The model under review builds one solid part; all positions refer to its coordinate system, in mm. A direction names the side the tool comes from. Coordinates: 2 decimals unless noted, no trailing zeros. Loops run counter-clockwise (first coordinate to the right, second up) from the corner with the lowest first, then second, coordinate; pieces in that order, holes last. Notation, with made-up numbers: M 9.5,-2.75 L 18.5,-2.75 A22 cw 18.5,34.25 Z; hole C 9,23 d4. An arc over 180 degrees is marked long. Return JSON: item names as keys, results as strings.
```python
from build123d import *

# Parameters (mm, degrees)
FLANGE_BASE1_START             = -5
FLANGE_BASE1_OUTLINE_W         = 35
FLANGE_BASE1_OUTLINE_H         = 80
FLANGE_BASE1_DEPTH             = 10
FURO_ROSCADO_DE_M10X1_51_D     = 8.5
FURO_ROSCADO_DE_M10X1_51_DEPTH = 29.946342369
FURO_ROSCADO_DE_M10X1_51_TIP   = 2.553657631
ESBO_O9_R                      = 10
CORTE_EXTRUS_O2_DEPTH          = 3
CORTE_EXTRUS_O3_DEPTH          = 45.218208919


# Read off the part's stored shape, not the designer's step: Flange-base1
with BuildPart() as part:
    # Flange-base1 outline → Flange-base1 (new body)
    with BuildSketch(Plane.XY.offset(FLANGE_BASE1_START)):
        Rectangle(FLANGE_BASE1_OUTLINE_W, FLANGE_BASE1_OUTLINE_H)
    extrude(amount=FLANGE_BASE1_DEPTH)

    # Furo roscado de M10x1.51
    with Locations(Plane.XY.offset(5)):
        with Locations((0, 25)):
            Hole(FURO_ROSCADO_DE_M10X1_51_D / 2, depth=FURO_ROSCADO_DE_M10X1_51_DEPTH)
            with Locations((0, 0, -(FURO_ROSCADO_DE_M10X1_51_DEPTH + FURO_ROSCADO_DE_M10X1_51_TIP / 2))):  # 118° drill point
                Cone(0, FURO_ROSCADO_DE_M10X1_51_D / 2, FURO_ROSCADO_DE_M10X1_51_TIP, mode=Mode.SUBTRACT)

    # Esboço9 → Corte-extrusão2 (cut)
    with BuildSketch(Plane.XY.offset(5)):
        with Locations((0, -15)):
            Circle(ESBO_O9_R)
    extrude(amount=-CORTE_EXTRUS_O2_DEPTH, mode=Mode.SUBTRACT)

    # Esboço10 → Corte-extrusão3 (cut, through all)
    with BuildSketch(Plane.XY.offset(2)):
        with BuildLine():
            Line((-6.5, -11.258342613), (-6.5, -18.741657387))
            ThreePointArc((-6.5, -18.741657387), (0, -22.5), (6.5, -18.741657387))
            Line((6.5, -18.741657387), (6.5, -11.258342613))
            ThreePointArc((6.5, -11.258342613), (0, -7.5), (-6.5, -11.258342613))
        make_face()
    extrude(amount=-CORTE_EXTRUS_O3_DEPTH, mode=Mode.SUBTRACT)


solid = part.part
```
1. Add section B-B on x = 0. Give the boundary of the cut face in (y, z).
Check values:
{"outline": "M -40,-5 L -22.5,-5 L -22.5,2 L -25,2 L -25,5 L -40,5 Z; M -7.5,-5 L 20.75,-5 L 20.75,5 L -5,5 L -5,2 L -7.5,2 Z; M 29.25,-5 L 40,-5 L 40,5 L 29.25,5 Z"}
2. Machinability: for faces 1 (the face through (-6.5, -15, -1)), 2 (the face through (7, -15, 2)), 3 (the face through (0, 1, 5)), which of the approach directions +Z, -Z, +X, -X, +Y, -Y give a long, thin tool a straight path to every point of the face, cutting with its end or side? Answer none if there is none.
Check values:
{"face 1": "+Z, -Z", "face 2": "+Z", "face 3": "+Z, +X, -X, +Y, -Y"}
3. Insertion check: pin 1 Ø18 at (x, y) = (0, -15) entering from +Z; pin 2 Ø5 at (x, y) = (0, 25) entering from +Z. Each pin has a flat end and moves straight along its axis. Give the tip position at first contact, or say it passes through.
Check values:
{"pin 1": "z = 2", "pin 2": "through"}
4. Add section D-D on x = -5. Give the boundary of the cut face in (y, z).
Check values:
{"outline": "M -40,-5 L -20.59,-5 L -20.59,2 L -23.66,2 L -23.66,5 L -40,5 Z; M -9.41,-5 L 40,-5 L 40,5 L -6.34,5 L -6.34,2 L -9.41,2 Z"}
5. The part is to be moulded in two halves that separate along X. For faces 4 (the face through (0, 40, 0)), 5 (the face through (17.5, -1, 0)), 6 (the face through (0.1, -7.5, -1.5)), 7 (the face through (-17.5, -1, 0)), say which applies: released by +X, released by -X, zero draft, split by the parting line, or undercut.
Check values:
{"face 4": "zero draft", "face 5": "released by +X", "face 6": "undercut", "face 7": "released by -X"}
6. Add section A-A on y = -15. Give the boundary of the cut face in (x, z), plus the area to 3 significant figures.
Check values:
{"outline": "M -17.5,-5 L -6.5,-5 L -6.5,2 L -10,2 L -10,5 L -17.5,5 Z; M 6.5,-5 L 17.5,-5 L 17.5,5 L 10,5 L 10,2 L 6.5,2 Z", "area": "199 mm²"}
7. To check wall thickness, follow line 1 (Y direction, x = 0, z = 2.5); line 2 (X direction, y = 25.5, z = -4); line 3 (X direction, y = -6, z = 4.5). State the ranges of each line that lie inside material, in increasing order.
Check values:
{"line 1": "-40 to -25, -5 to 20.75, 29.25 to 40", "line 2": "-17.5 to -4.22, 4.22 to 17.5", "line 3": "-17.5 to -4.36, 4.36 to 17.5"}
8. Add section C-C on z = 3. Give the boundary of the cut face in (x, y).
Check values:
{"outline": "M -17.5,-40 L 17.5,-40 L 17.5,40 L -17.5,40 Z; hole C 0,-15 d20; hole C 0,25 d8.5"}
